Read the model definition and answer for the solid it produces. Units are mm, in the model's axes. A direction names the side the tool comes from. Coordinates: 2 decimals unless noted, no trailing zeros. Write each loop counter-clockwise with the first axis right and the second up, starting at its lowest first coordinate (ties: lowest second). Pieces come first, ordered by that corner, then holes. Notation, with made-up numbers: M -18.75,-20.5 L 1.25,-20.5 A33 ccw 1.25,13.5 Z; hole C 59.25,47.5 d5. An arc over 180 degrees is marked long. Write item = value, one per line.
from build123d import *

# Parameters (mm, degrees)
EXTRUDE_1_DEPTH          = 4
CUT_EXTRUDE_1_DEPTH      = 38.905694823
CUT_EXTRUDE_1_DEPTH_BACK = 38.905694823
SKETCH_2_R               = 1
SKETCH_3_W               = 14
SKETCH_3_H               = 20.72
CUT_EXTRUDE_3_DEPTH      = 3
SKETCH_5_W               = 5
SKETCH_5_H               = 20.72
CUT_EXTRUDE_4_DEPTH      = 4
SKETCH_13_W              = 24.72
SKETCH_13_H              = 4
EXTRUDE_5_DEPTH          = 30
SKETCH_15_R              = 10
EXTRUDE_6_DEPTH          = 4
SKETCH_14_R              = 1.25
CUT_EXTRUDE_7_DEPTH      = 4
FILLET_1_R               = 10
FILLET_2_R               = 10
SKETCH_6_R               = 11
CUT_EXTRUDE_9_DEPTH      = 4
SKETCH_17_W              = 24.72
SKETCH_17_H              = 4
CUT_EXTRUDE_10_DEPTH     = 16
FILLET_3_R               = 2
FILLET_4_R               = 2
FILLET_5_R               = 2
FILLET_6_R               = 2
SKETCH_18_R              = 3
CUT_EXTRUDE_11_DEPTH     = 13


with BuildPart() as part:
    # 草图1 → 凸台-拉伸1 (new body)
    with BuildSketch(Plane(origin=(0, 0, 0), x_dir=(1, 0, 0), z_dir=(0, 1, 0))):
        with BuildLine():
            Line((6.61, -12.36), (9.61, -12.36))
            Line((9.61, -12.36), (9.61, -9.36))
            Line((9.61, -9.36), (9.61, 9.36))
            Line((9.61, 9.36), (9.61, 12.36))
            Line((9.61, 12.36), (6.61, 12.36))
            Line((6.61, 12.36), (-32.61, 12.36))
            ThreePointArc((-32.61, 12.36), (-34.731320344, 11.481320344), (-35.61, 9.36))
            Line((-35.61, 9.36), (-35.61, -9.36))
            ThreePointArc((-35.61, -9.36), (-34.731320344, -11.481320344), (-32.61, -12.36))
            Line((-32.61, -12.36), (6.61, -12.36))
        make_face()
    extrude(amount=EXTRUDE_1_DEPTH)

    # 草图2 → 切除-拉伸1 (cut, two sides: drawn at the far end of the back side and taken through both)
    with BuildSketch(Plane(origin=(0, 0, 0), x_dir=(1, 0, 0), z_dir=(0, 1, 0)).offset(-CUT_EXTRUDE_1_DEPTH_BACK)):
        with Locations(Location((7.25, -10.25, 0), (0, 0, 270))):
            Circle(SKETCH_2_R)
        with Locations(Location((7.25, 10.25, 0), (0, 0, 270))):
            Circle(SKETCH_2_R)
        with Locations(Location((-17.2, -10.25, 0), (0, 0, 270))):
            Circle(SKETCH_2_R)
        with Locations(Location((-17.2, 10.25, 0), (0, 0, 270))):
            Circle(SKETCH_2_R)
    extrude(amount=CUT_EXTRUDE_1_DEPTH + CUT_EXTRUDE_1_DEPTH_BACK, mode=Mode.SUBTRACT)

    # 草图3 → 切除-拉伸3 (cut)
    with BuildSketch(Plane(origin=(0, 4, 0), x_dir=(1, 0, 0), z_dir=(0, 1, 0))):
        with Locations((-1.39, 0)):
            Rectangle(SKETCH_3_W, SKETCH_3_H)
    extrude(amount=-CUT_EXTRUDE_3_DEPTH, mode=Mode.SUBTRACT)

    # 草图5 → 切除-拉伸4 (cut)
    with BuildSketch(Plane(origin=(0, 4, 0), x_dir=(1, 0, 0), z_dir=(0, 1, 0))):
        with Locations((-10.89, 0)):
            Rectangle(SKETCH_5_W, SKETCH_5_H)
    extrude(amount=-CUT_EXTRUDE_4_DEPTH, mode=Mode.SUBTRACT)

    # 草图13 → 凸台-拉伸5 (add)
    with BuildSketch(Plane(origin=(9.61, 0, 0), x_dir=(0, 0, -1), z_dir=(1, 0, 0))):
        with Locations((0, 2)):
            Rectangle(SKETCH_13_W, SKETCH_13_H)
    extrude(amount=EXTRUDE_5_DEPTH)

    # 草图15 → 凸台-拉伸6 (add)
    with BuildSketch(Plane(origin=(0, 4, 0), x_dir=(1, 0, 0), z_dir=(0, 1, 0))):
        with Locations(Location((27.25, 0, 0), (0, 0, 270))):
            Circle(SKETCH_15_R)
    extrude(amount=EXTRUDE_6_DEPTH)

    # 草图14 → 切除-拉伸7 (cut, symmetric)
    with BuildSketch(Plane(origin=(0, 4, 0), x_dir=(1, 0, 0), z_dir=(0, 1, 0))):
        with Locations(Location((27.25, -7, 0), (0, 0, 270))):
            Circle(SKETCH_14_R)
        with Locations(Location((34.25, 0, 0), (0, 0, 270))):
            Circle(SKETCH_14_R)
        with Locations(Location((27.25, 7, 0), (0, 0, 270))):
            Circle(SKETCH_14_R)
        with Locations(Location((20.25, 0, 0), (0, 0, 270))):
            Circle(SKETCH_14_R)
    extrude(amount=CUT_EXTRUDE_7_DEPTH, both=True, mode=Mode.SUBTRACT)

    # 圆角1
    fillet_1_edges = [part.edges().sort_by_distance(p)[0] for p in [
        (39.61, 2, -12.36),
    ]]
    fillet(fillet_1_edges, radius=FILLET_1_R)

    # 圆角2
    fillet_2_edges = [part.edges().sort_by_distance(p)[0] for p in [
        (39.61, 2, 12.36),
    ]]
    fillet(fillet_2_edges, radius=FILLET_2_R)

    # 草图6 → 切除-拉伸9 (cut)
    with BuildSketch(Plane(origin=(0, 4, 0), x_dir=(1, 0, 0), z_dir=(0, 1, 0))):
        with Locations((-25.5, 0)):
            Circle(SKETCH_6_R)
    extrude(amount=-CUT_EXTRUDE_9_DEPTH, mode=Mode.SUBTRACT)

    # 草图17 → 切除-拉伸10 (cut)
    with BuildSketch(Plane.ZY.offset(35.61)):
        with Locations((0, 2)):
            Rectangle(SKETCH_17_W, SKETCH_17_H)
    extrude(amount=-CUT_EXTRUDE_10_DEPTH, mode=Mode.SUBTRACT)

    # 圆角3
    fillet_3_edges = [part.edges().sort_by_distance(p)[0] for p in [
        (-19.61, 2, 12.36),
    ]]
    fillet(fillet_3_edges, radius=FILLET_3_R)

    # 圆角4
    fillet_4_edges = [part.edges().sort_by_distance(p)[0] for p in [
        (-19.61, 2, -12.36),
    ]]
    fillet(fillet_4_edges, radius=FILLET_4_R)

    # 圆角5
    fillet_5_edges = [part.edges().sort_by_distance(p)[0] for p in [
        (-19.61, 2, -9.290204519),
    ]]
    fillet(fillet_5_edges, radius=FILLET_5_R)

    # 圆角6
    fillet_6_edges = [part.edges().sort_by_distance(p)[0] for p in [
        (-19.61, 2, 9.290204519),
    ]]
    fillet(fillet_6_edges, radius=FILLET_6_R)

    # 草图18 → 切除-拉伸11 (cut)
    with BuildSketch(Plane(origin=(0, 8, 0), x_dir=(1, 0, 0), z_dir=(0, 1, 0))):
        with Locations(Location((27.25, 0, 0), (0, 0, 270))):
            Circle(SKETCH_18_R)
    extrude(amount=-CUT_EXTRUDE_11_DEPTH, mode=Mode.SUBTRACT)


solid = part.part
Item 1: Find section D-D (x = 34.25). Determine the outline of the cut face in (y, z), and give its area (3 significant figures).
Worked answers:
outline = M 0,-11.22 L 4,-11.22 L 4,-7.14 L 8,-7.14 L 8,-1.25 L 0,-1.25 Z; M 0,1.25 L 8,1.25 L 8,7.14 L 4,7.14 L 4,11.22 L 0,11.22 Z
area = 127 mm²
Item 2: Consider line 1 along X through (y, z) = (5.05, 0); line 2 along X through (y, z) = (2, 0); line 3 along Z through (x, y) = (-6.5, 2). Determine where each line is inside the solid, lowest interval first. Write a range as from..to.
Worked answers:
line_1 = 17.25..19, 21.5..24.25, 30.25..33, 35.5..37.25
line_2 = -14.5..-13.39, 5.61..19, 21.5..24.25, 30.25..33, 35.5..39.61
line_3 = -12.36..-10.36, 10.36..12.36
Item 3: Find section C-C (x = 7.25). Determine the outline of the cut face in (y, z), and give its area (3 significant figures).
Worked answers:
outline = M 0,-12.36 L 4,-12.36 L 4,-11.25 L 0,-11.25 Z; M 0,-9.25 L 4,-9.25 L 4,9.25 L 0,9.25 Z; M 0,11.25 L 4,11.25 L 4,12.36 L 0,12.36 Z
area = 82.9 mm²
Item 4: Which of the six approach directions +Z, -Z, +X, -X, +Y, -Y give full straight-line access (tool end or side, diameter ignored) to faces 4 (the face through (-8.39, 0.5, 0.1)), 5 (the face through (-19, 2, 11.8)), 6 (the face through (-19.41, 2.03, -9.46)), 7 (the face through (-4, 2, 10.36))?
Worked answers:
face_4 = +Y, -Y
face_5 = +Z, -X, +Y, -Y
face_6 = -X, +Y, -Y
face_7 = +Y
Item 5: Find section A-A (y = 2.75). State how many separate pieces and enclosed holes the cut face has, and give its area (3 significant figures).
Worked answers:
separate_pieces = 1
enclosed_holes = 10
area = 898 mm²
Item 6: Flat-ended cylindrical pins translate along their axes: pin 1 (2 mm diameter, centred on x = 27.25, z = 7, fed in from +Y); pin 2 (1 mm diameter, centred on y = 2.5, z = -9, fed in from -X); pin 3 (3.5 mm diameter, centred on y = 2.5, z = 3, fed in from -X); pin 4 (11 mm diameter, centred on x = -1.5, z = 0, fed in from +Y). Find the tip coordinate at first contact, or state that the pin passes through.
Worked answers:
pin_1 = through
pin_2 = -19.43
pin_3 = -15.58
pin_4 = 1
Item 7: Find section B-B (z = 0). Determine the outline of the cut face in (x, y).
Worked answers:
outline = M -14.5,0 L -13.39,0 L -13.39,4 L -14.5,4 Z; M -8.39,0 L 19,0 L 19,8 L 17.25,8 L 17.25,4 L 5.61,4 L 5.61,1 L -8.39,1 Z; M 21.5,0 L 24.25,0 L 24.25,8 L 21.5,8 Z; M 30.25,0 L 33,0 L 33,8 L 30.25,8 Z; M 35.5,0 L 39.61,0 L 39.61,4 L 37.25,4 L 37.25,8 L 35.5,8 Z
Item 8: For a pull along X with two mould halves and no side action, classify faces 1 (the face through (6, 2, -12.36)), 2 (the face through (-19.397, 2.028, 9.434)), 3 (the face through (-13.39, 2, 0)) as released by +X, released by -X, zero draft, split by the parting line, or undercut.
Worked answers:
face_1 = zero draft
face_2 = released by -X
face_3 = undercut
